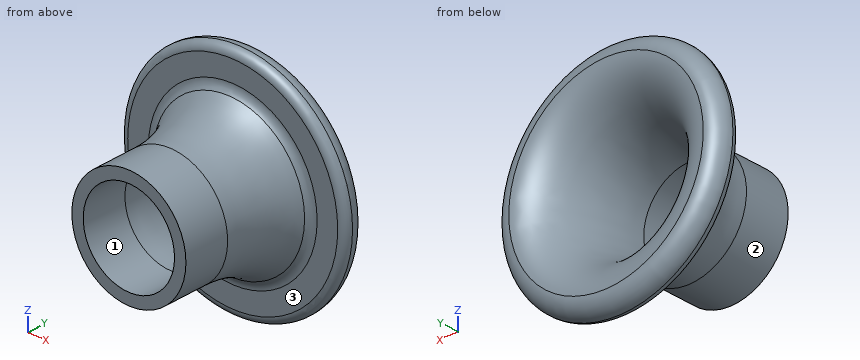
```python
from build123d import *


with BuildPart() as f1:
    # F0 (on Top) → F1 (revolve)
    with BuildSketch(Plane.XY):
        with BuildLine():
            ThreePointArc((29.21, 18.923), (30.7366435406, 19.5553564594), (31.369, 21.082))
            ThreePointArc((31.369, 21.082), (30.1042870812, 24.1352870812), (27.051, 25.4))
            add(Edge.make_bspline(
                [(27.051, 25.4), (12.7, 25.4), (12.7, 0)],
                knots=[0, 0, 0, 1.5707963268, 1.5707963268, 1.5707963268], degree=2, weights=[1, 0.7071067812, 1]))
            Line((12.7, 0), (12.7, -12.7))
            Line((12.7, -12.7), (15.875, -12.7))
            Line((15.875, -12.7), (15.875, 0))
            add(Edge.make_bspline(
                [(21.0444702233, 17.778371929), (15.875, 11.5635524722), (15.875, 0)],
                knots=[0.5674091227, 0.5674091227, 0.5674091227, 1.5707963268, 1.5707963268, 1.5707963268], degree=2, weights=[1, 0.8767693476, 1]))
            ThreePointArc((21.0444702233, 17.778371929), (22.1374182752, 18.6226352703), (23.485415702, 18.923))
            Line((23.485415702, 18.923), (29.21, 18.923))
        make_face()
    revolve(axis=Axis((0, 35.1700206795, 0), (0, 1, 0)))


solid = f1.part
```
Read the model definition and answer for the solid it produces. Units are mm, in the model's axes. Face numbers are marked on the shaded views. Give positions to 0.01 mm unless a question says otherwise; leave off trailing zeros. Write each loop counter-clockwise with the first axis right and the second up, starting at its lowest first coordinate (ties: lowest second). Pieces come first, ordered by that corner, then holes. Notation, with made-up numbers: (35.5, -11.5) -> (87.5, -11.5) arc R35 ccw to (87.5, 26.5) -> close; hole circle Ø9 at (71, 55.5). An arc over 180 degrees is marked (long way). Answer as a JSON object with one key per item and string values.
1) For a pull along Z with two mould halves and no side action, classify the marked faces 1, 2 and 3 as pulls with the +Z half, pulls with the -Z half, needs draft (parallel to the pull), parting line crosses it, or undercut.
Findings below:
{"face 1": "undercut", "face 2": "parting line crosses it", "face 3": "needs draft"}
2) Section A-A on y = -7.5 is taken. Write down the section's boundary in (x, z) (3 decimals).
Findings below:
{"outline": "circle Ø31.75 at (0, 0); hole circle Ø25.4 at (0, 0)"}
3) Flat-ended cylindrical pins translate along their axes: pin 1 Ø10 at (y, z) = (9.5, 1) entering from +X; pin 2 Ø4 at (y, z) = (19.5, -21) entering from -X; pin 3 Ø2 at (x, y) = (-12, 18.5) entering from -Z; pin 4 Ø17.5 at (x, z) = (2, -5.5) entering from -Y. Find the tip coordinate at first contact, or state that the pin passes through.
Findings below:
{"pin 1": "stops at x = 18.92", "pin 2": "stops at x = -24.66", "pin 3": "stops at z = -28.31", "pin 4": "stops at y = -12.7"}
4) Straight lines are drawn through the part: probe 1 along Z at (x, y) = (0, -4) (3 decimals); probe 2 along X at (y, z) = (11, 2). For each, find the intervals that lie inside material, in ascending order. Write a range as from..to.
Findings below:
{"probe 1": "z = -15.875..-12.7, 12.7..15.875", "probe 2": "x = -17.4..-13.97, 13.97..17.4"}
